Check sheet for the modelled part. Datum: model origin and axes. Units: mm. Round coordinates to 2 decimals unless told otherwise and drop trailing zeros. Loops run counter-clockwise (first coordinate to the right, second up) from the corner with the lowest first, then second, coordinate; pieces in that order, holes last. Notation, with made-up numbers: (-7, -17.5) - (14, -17.5) arc R21 ccw to (14, -4.5) - close; hole circle Ø1 at (-23, 58). An arc over 180 degrees is marked (long way). Return JSON: item names as keys, results as strings.
Autodesk Inventor part; units mm, degrees
ref_plane "Start Plane" through (0, 0, 0) normal (0, 0, 1) x (1, 0, 0)
ref_plane "End Plane" through (0, 0, 525) normal (0, 0, 1) x (1, 0, 0)
ref_plane "Work Plane4" through (0, -20, 525) normal (0, 0, 1) x (1, 0, 0)
ref_plane "Start Plane" through (0, 0, 0) normal (0, 0, 1) x (1, 0, 0)
ref_plane "End Plane" through (0, 0, 525) normal (0, 0, 1) x (1, 0, 0)
sketch "Sketch" plane through (0, 0, 0) normal (0, 0, 1) x (1, 0, 0)
  line L0 (-25, -21) -> (-25, 21)
  line L1 (-21, 25) -> (21, 25)
  line L2 (25, 21) -> (25, -21)
  line L3 (21, -25) -> (-21, -25)
  arc A0 (-25, -21) -> (-21, -25) centre (-21, -21) ccw
  arc A1 (25, 21) -> (21, 25) centre (21, 21) ccw
  arc A2 (-21, 25) -> (-25, 21) centre (-21, 21) ccw
  arc A3 (21, -25) -> (25, -21) centre (21, -21) ccw
  arc A4 (-21, 23) -> (-23, 21) centre (-21, 21) ccw
  line L4 (-21, 23) -> (21, 23)
  arc A5 (23, 21) -> (21, 23) centre (21, 21) ccw
  line L5 (23, 21) -> (23, -21)
  arc A6 (21, -23) -> (23, -21) centre (21, -21) ccw
  line L6 (21, -23) -> (-21, -23)
  arc A7 (-23, -21) -> (-21, -23) centre (-21, -21) ccw
  line L7 (-23, -21) -> (-23, 21)
  line L8 (0, 36.1598) -> (0, -36.1598) construction
  line L9 (-36.1598, 0) -> (36.1598, 0) construction
  dimension "d7" = 4
  dimension "d9" = 50
  dimension "d11" = 50
  dimension "d12" = 2
  dimension "d15" = 25
  dimension "d16" = 25
extrude "Body" add sketch "Sketch" along normal up to surface (525 mm away) from surface at 0
sketch "Sketch3" plane through (0, 0, 0) normal (0, 0, 1) x (1, 0, 0)
  line L0 (0, 0) -> (10, 0)
ref_plane "Work Plane3" through (0, 0, 0) normal (0, -1, 0) x (1, 0, 0)
sketch "Sketch4" plane through (0, 0, 0) normal (0, -1, 0) x (1, 0, 0)
  line L0 (-2, 0) -> (12, 0)
  line L1 (-2, 525) -> (12, 525)
  dimension "d18" = 525
ref_plane "Work Plane4" through (0, -20, 525) normal (0, 0, 1) x (1, 0, 0)
split "Split1" plane through (0, -20, 525) removes the side toward (0, 0, 1)
sketch "Sketch5" plane through (21, 25, 525) normal (0, 1, 0) x (1, 0, 0)
  line L0 (-42, 0) -> (0, 0)
  line L1 (0, 525) -> (0, 0)
  line L2 (-42, 525) -> (0, 525)
  line L3 (-42, 525) -> (-42, 0)
  line L4 (-42, 0) -> (0, 0)
  line L5 (-21, 0) -> (-21, 21.8701)
  line L6 (-37, 32) -> (-5, 32)
  line L7 (-5, 32) -> (-5, 68)
  line L8 (-5, 68) -> (-37, 68)
  line L9 (-37, 68) -> (-37, 32)
  point P0 (-21, 525)
  dimension "d19" = 32
  dimension "d20" = 36
  dimension "d21" = 32
hole "Hole1" at (-16, 25, 457) at (-16, 25, 493) at (16, 25, 493) at (16, 25, 457) direction (0, -1, 0) diameter 5 depth 50
equation "\"d7\" = G_IR"
equation "\"d9\" = G_W"
equation "\"d11\" = G_H"
equation "\"d12\" = G_T"
equation "\"d15\" = 0.5 * d9"
equation "\"d16\" = 0.5 * d11"
equation "\"d3\" = G_L"
equation "\"G_W\" = 50"
equation "\"G_H\" = 50"
equation "\"G_T\" = 2"
equation "\"G_IR\" = 4"
equation "\"G_L\" = d18"
equation "\"G_OFFSET_START\" = 0"
equation "\"G_OFFSET_END\" = -25"
equation "\"d14\" = G_OFFSET_END + B_L"
properties part number "ISO 10799-2 - 50x50x2 - 525" material "Steel, Galvanized"
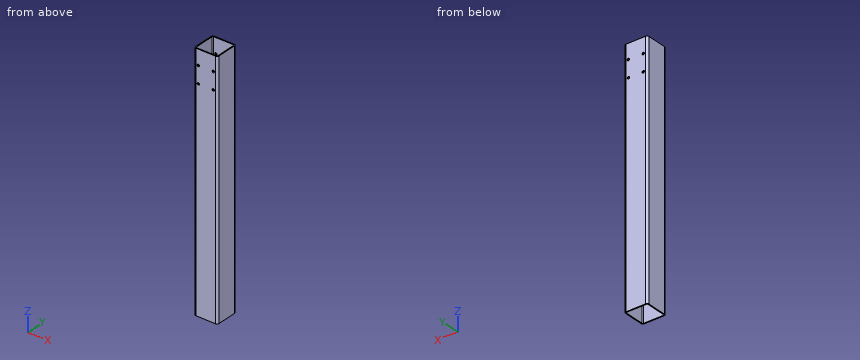
Q1. Depth check by flat-ended pin: P1, Ø6, axis at x = 16, z = 493, coming from the -Y side; P2, Ø3, axis at x = -16, z = 493, coming from the +Y side (3 decimals). Enter the tip coordinate at first touch or a pass-through.
Answer key:
{"P1": "stops at y = -25", "P2": "passes through"}
Q2. Scan lines: probe 1 along Z at (x, y) = (16, -24.1); probe 2 along Y at (x, z) = (12.5, 471). Record each from-to range of solid material in increasing order. Write a range as [from, to].
Answer key:
{"probe 1": "z = [0, 454.5], [459.5, 490.5], [495.5, 525]", "probe 2": "y = [-25, -23], [23, 25]"}
Q3. Sectioned sample at A-A (y = -6). Enter the section's corners in (x, z), plus the area to 3 significant figures.
Answer key:
{"outline": "(-25, 0) - (-23, 0) - (-23, 525) - (-25, 525) - close; (23, 0) - (25, 0) - (25, 525) - (23, 525) - close", "area": "2,100 mm²"}
Q4. Sectioned sample at B-B (z = 334.5). Enter the section's corners in (x, y).
Answer key:
{"outline": "(-25, -21) arc R4 ccw to (-21, -25) - (21, -25) arc R4 ccw to (25, -21) - (25, 21) arc R4 ccw to (21, 25) - (-21, 25) arc R4 ccw to (-25, 21) - close; hole (-23, -21) arc R2 ccw to (-21, -23) - (21, -23) arc R2 ccw to (23, -21) - (23, 21) arc R2 ccw to (21, 23) - (-21, 23) arc R2 ccw to (-23, 21) - close"}
